Could you check a few things on this model? Use its own coordinates, in mm. A direction names the side the tool comes from. Coordinates: 2 decimals unless noted, no trailing zeros. Loops run counter-clockwise (first coordinate to the right, second up) from the corner with the lowest first, then second, coordinate; pieces in that order, holes last.
from build123d import *

# Parameters (mm, degrees)
F0_R        = 44.45
F1_DEPTH    = 76.2
F3_DEPTH    = 38.1
F4_T1_DEPTH = 56.0791508125
F5_DEPTH    = 76.201


# Not quite as in the source:
# - a fillet or chamfer that OpenCascade refuses, or shapes differently, is made with other operations: its cross-section is extruded or revolved along the edge and cut away or added


with BuildPart() as f1:
    # F0 (on Top) → F1 (new body)
    with BuildSketch(Plane.XY):
        Circle(F0_R)
    extrude(amount=F1_DEPTH)

    # F2 (on face) → F3 (cut)
    with BuildSketch(Plane.XY.offset(76.2)):
        with BuildLine():
            Line((0, 28.575), (0, 38.1))
            ThreePointArc((0, 38.1), (-28.175329967, 20.986026826), (-25.976370723, -11.90625))
            ThreePointArc((-25.976370723, -11.90625), (-24.0494461345, 15.4322637881), (0, 28.575))
        make_face()
        with BuildLine():
            ThreePointArc((0, 28.575), (-24.0494461345, 15.4322637881), (-25.976370723, -11.90625))
            ThreePointArc((-25.976370723, -11.90625), (-14.636026826, -21.825329967), (0, -25.4))
            ThreePointArc((0, -25.4), (-25.4, 0), (0, 25.4))
            Line((0, 25.4), (0, 28.575))
        make_face()
        with BuildLine():
            ThreePointArc((0, 25.4), (-25.4, 0), (0, -25.4))
            Line((0, -25.4), (0, -2.38125))
            ThreePointArc((0, -2.38125), (-2.38125, 0), (0, 2.38125))
            Line((0, 2.38125), (0, 25.4))
        make_face()
        with BuildLine():
            Line((0, -2.38125), (0, -25.4))
            ThreePointArc((0, -25.4), (17.9605122421, -17.9605122421), (25.4, 0))
            ThreePointArc((25.4, 0), (17.9605122421, 17.9605122421), (0, 25.4))
            Line((0, 25.4), (0, 2.38125))
            ThreePointArc((0, 2.38125), (1.6837980227, 1.6837980227), (2.38125, 0))
            ThreePointArc((2.38125, 0), (1.6837980227, -1.6837980227), (0, -2.38125))
        make_face()
        with BuildLine():
            Line((28.575, 0), (38.1, 0))
            ThreePointArc((38.1, 0), (26.9407683632, 26.9407683632), (0, 38.1))
            Line((0, 38.1), (0, 28.575))
            ThreePointArc((0, 28.575), (20.2055762724, 20.2055762724), (28.575, 0))
        make_face()
    extrude(amount=-F3_DEPTH, mode=Mode.SUBTRACT)

    # F4: chamfer of 6.35 x 2.3112109876 on 1 edges, made by hand

    # F4_s2 → F4_t1 (cut)
    with BuildSketch(Plane.XY.offset(38.1)):
        with BuildLine():
            Line((0, 25.4845857979), (6.9087994087, 27.7272269751))
            ThreePointArc((6.9087994087, 27.7272269751), (3.5951834098, 28.3479325745), (0, 28.575))
            Line((0, 28.575), (0, 25.4845857979))
        make_face()
    extrude(amount=F4_T1_DEPTH, mode=Mode.SUBTRACT)

    # F5 (cut, through all): a face of the model
    f5_faces = [f1.faces().sort_by_distance(p)[0] for p in [
        (0, 0, 76.2),
    ]]
    extrude(f5_faces, amount=-F5_DEPTH, mode=Mode.SUBTRACT)


solid = f1.part
(1) Which directions (+Z, -Z, +X, -X, +Y, -Y) give clear straight access to the entire face, cutting with the end or side of a thin tool? Please do faces 4 (the face through (-31.742, 7.048, 57.417)), 5 (the face through (19, -19, 76.2)).
Answers:
face 4: +Z
face 5: +Z, +X, -X, +Y, -Y
(2) Imagine slicing it at C-C, the plane x = 31. Write out the boundary of the cut face in (y, z), and give its area (3 significant figures).
Answers:
outline: (-31.86, 0) - (31.86, 0) - (31.86, 76.2) - (22.15, 76.2) - (22.15, 38.1) - (0, 38.1) - (0, 76.2) - (-31.86, 76.2) - close
area: 4,010 mm2
(3) Imagine slicing it at A-A, the plane z = 62. Write out the boundary of the cut face in (x, y) (3 decimals), and give its area (3 significant figures).
Answers:
outline: circle Ø88.9 at (0, 0); hole (0, -25.4) arc R25.4 ccw to (0, 25.4) - (0, 25.485) - (6.909, 27.727) arc R28.575 cw to (28.575, 0) - (38.1, 0) arc R38.1 ccw to (0, 38.1) arc R31.75 ccw to start
area: 3,100 mm2
(4) I need wall thicknesses on probe 1 along Y at (x, z) = (0, 22); probe 2 along Y at (x, z) = (9, 43); probe 3 along X at (y, z) = (18.5, 58.5). Which ranges of each line are inside material? Lowest first, please.
Answers:
probe 1: y = -44.45 to -2.38, 2.38 to 44.45
probe 2: y = -43.53 to -23.75, 23.75 to 27.12, 37.02 to 43.53
probe 3: x = -40.42 to -29.33, 17.4 to 21.78, 33.31 to 40.42
(5) We'd pull the mould along X, two halves only. Please class faces 1 (the face through (42.397, 13.352, 37.567)), 2 (the face through (22.352, 17.803, 57.417)), 3 (the face through (-1, -9, 0)): +X half, -X half, draft (parallel to the pull), parting line (faces both ways), or undercut.
Answers:
face 1: parting line
face 2: undercut
face 3: draft
(6) For pin 1 (12 mm diameter, centred on y = -32, z = 57, fed in from +X); pin 2 (8 mm diameter, centred on y = -22.5, z = 11.5, fed in from +X); pin 3 (10.5 mm diameter, centred on x = 34.5, z = 48, fed in from +Y), each with a flat end and sliding along its axis, tell me the tip position at first contact or that it passes through.
Answers:
pin 1: stops at x = 36.05
pin 2: stops at x = 40.42
pin 3: stops at y = 33.47
(7) Imagine slicing it at D-D, the plane x = 13. Write out the boundary of the cut face in (y, z), and give its area (3 significant figures).
Answers:
outline: (-42.51, 0) - (42.51, 0) - (42.51, 76.2) - (35.81, 76.2) - (35.81, 38.1) - (25.45, 38.1) - (25.45, 76.2) - (21.82, 76.2) - (21.82, 38.1) - (-21.82, 38.1) - (-21.82, 76.2) - (-42.51, 76.2) - close
area: 4,420 mm2
(8) Imagine slicing it at B-B, the plane y = -12. Write out the boundary of the cut face in (x, z).
Answers:
outline: (-42.8, 0) - (42.8, 0) - (42.8, 76.2) - (22.39, 76.2) - (22.39, 38.1) - (-25.91, 38.1) - (-25.91, 76.2) - (-42.8, 76.2) - close
